Could you check a few things on this model? Use its own coordinates, in mm. Face numbers are marked on the shaded views. A direction names the side the tool comes from. Round coordinates to 2 decimals unless told otherwise and drop trailing zeros. Loops run counter-clockwise (first coordinate to the right, second up) from the corner with the lowest first, then second, coordinate; pieces in that order, holes last. Notation, with made-up numbers: (65.25, 50) -> (90.25, 50) arc R29 cw to (90.25, 71) -> close; hole circle Ø4 at (83, 85.25). An arc over 180 degrees is marked (long way). One line per item, written item: value.
Autodesk Inventor part; units mm, degrees
ref_plane "YZ Plane" through (0, 0, 0) normal (1, 0, 0) x (0, 1, 0)
ref_plane "XZ Plane" through (0, 0, 0) normal (0, 1, 0) x (-1, 0, 0)
ref_plane "XY Plane" through (0, 0, 0) normal (0, 0, 1) x (1, 0, 0)
sketch "Sketch1" plane through (0, 0, 0) normal (0, 1, 0) x (-1, 0, 0)
  line L0 (22.75, -10.36) -> (7.75, -10.36)
  line L1 (7.75, -10.36) -> (-0.1031, 0)
  circle A0 centre (4.34, -10.36) radius 1
  line L2 (22.75, 10.36) -> (7.75, 10.36)
  circle A1 centre (12.64, 0) radius 9.6 construction
  line L3 (22.75, 12.36) -> (22.75, -12.36)
  circle A2 centre (4.34, 10.36) radius 1
  line L4 (7.75, 10.36) -> (-0.1031, 0)
  line L5 (26.25, 17) -> (26.25, -17)
  line L6 (22.75, -12.36) -> (-22.75, -12.36)
  line L7 (22.75, 0) -> (-22.75, 0) construction
  line L8 (26.25, -17) -> (-28.75, -17)
  line L9 (26.25, -17) -> (-28.75, 17) construction
  line L10 (-28.75, -17) -> (26.25, 17) construction
  line L11 (-22.75, 12.36) -> (22.75, 12.36)
  line L12 (-28.75, 17) -> (26.25, 17)
  line L13 (-28.75, -17) -> (-28.75, 17)
  circle A3 centre (-16.36, 10.25) radius 1
  line L14 (-22.75, -12.36) -> (-22.75, 12.36)
  circle A4 centre (-16.36, -10.25) radius 1
  point P0 (0, 0)
  point P1 (-1.25, 0)
  point P2 (0, 0)
  point P3 (22.75, -10.36)
  dimension "d0" = 55
  dimension "d1" = 34
  dimension "d2" = 45.5
  dimension "d3" = 24.72
  dimension "d4" = 2
  dimension "d6" = 18.41
  dimension "d7" = 20.5
  dimension "d8" = 19.2
  dimension "d9" = 10.11
  dimension "d10" = 13
  dimension "d11" = 15
  dimension "d12" = 3.5
  dimension "d13" = 2
  dimension "d14" = 3.41
  dimension "d51" = 20.7
extrude "Extrusion1" add sketch "Sketch1" along normal mid plane 1 contours L3 L6 L14 L11 L2 L4 L1 L0 | L5 L8 L13 L12
extrude "Extrusion2" add sketch "Sketch1" along normal blind 35 contours L5 L8 L13 L12
fillet "Fillet1" radius 3 8 edges at (1.25, -0.5, -17) (28.75, -0.5, 0) (1.25, -0.5, 17) (-26.25, -0.5, 0) (28.75, 17.25, -17) (28.75, 17.25, 17) (-26.25, 17.25, 17) (-26.25, 17.25, -17)
sketch "Sketch3" plane through (-23.25, 35, 17) normal (0, 0, 1) x (1, 0, 0)
  line L0 (46, -34.5) -> (46, 0)
  circle A0 centre (46, -28) radius 1.5
  line L1 (49, -32.5) -> (0, -32.5)
  circle A1 centre (46, -17) radius 1.5
  circle A2 centre (46, -6) radius 1.5
  circle A3 centre (30, -28) radius 1.5
  circle A4 centre (30, -17) radius 1.5
  circle A5 centre (30, -6) radius 1.5
  line L2 (52, -32.5) -> (52, 0)
  point P0 (23.25, -35)
  dimension "d20" = 3
  dimension "d23" = 11
  dimension "d26" = 16
  dimension "d29" = 4.5
  dimension "d37" = 6
hole "Hole1" at (22.75, 7, 17) at (6.75, 7, 17) at (6.75, 18, 17) at (22.75, 18, 17) at (22.75, 29, 17) at (6.75, 29, 17) direction (0, 0, -1) diameter 2.459 depth 3 tip angle 118 counterbore diameter 3.9 counterbore depth 1.8
properties part number "basket"
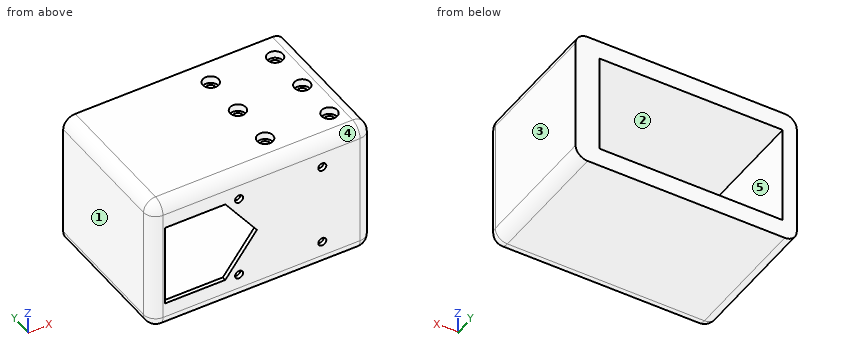
(1) If we section it at C-C, the plane x = -4: Please give me the cut outline in (y, z), then the cut area to 3 significant figures.
Recorded:
outline: (-0.5, -14) arc R3 ccw to (2.5, -17) -> (35, -17) -> (35, -12.36) -> (0.5, -12.36) -> (0.5, -11.3) -> (-0.5, -11.3) -> close; (-0.5, -9.42) -> (0.5, -9.42) -> (0.5, -5.41) -> (-0.5, -5.41) -> close; (-0.5, 5.41) -> (0.5, 5.41) -> (0.5, 9.42) -> (-0.5, 9.42) -> close; (-0.5, 11.3) -> (0.5, 11.3) -> (0.5, 12.36) -> (35, 12.36) -> (35, 17) -> (2.5, 17) arc R3 ccw to (-0.5, 14) -> close
area: 336 mm²
(2) If we section it at A-A, the plane x = -10: Please give me the cut outline in (y, z), then the cut area to 3 significant figures.
Recorded:
outline: (-0.5, -14) arc R3 ccw to (2.5, -17) -> (35, -17) -> (35, -12.36) -> (0.5, -12.36) -> (0.5, -10.36) -> (-0.5, -10.36) -> close; (-0.5, 10.36) -> (0.5, 10.36) -> (0.5, 12.36) -> (35, 12.36) -> (35, 17) -> (2.5, 17) arc R3 ccw to (-0.5, 14) -> close
area: 330 mm²
(3) Thinking about a two-plate mould opening in Z: for the marked faces 3, 4 and 5, which applies, released by +Z, released by -Z, zero draft, split by the parting line, or undercut?
Recorded:
face 3: zero draft
face 4: released by +Z
face 5: undercut
(4) I'm going to push a flat-ended pin straight in: pin 1 Ø3.5 at (x, y) = (22.75, 18) entering from +Z. Where does the tip first touch, or does it pass through?
Recorded:
pin 1: z = 15.2
(5) If we section it at B-B, the plane y = 10.5: Please give me the cut outline in (x, z).
Recorded:
outline: (-26.25, -14) arc R3 ccw to (-23.25, -17) -> (25.75, -17) arc R3 ccw to (28.75, -14) -> (28.75, 14) arc R3 ccw to (25.75, 17) -> (-23.25, 17) arc R3 ccw to (-26.25, 14) -> close; hole (-22.75, -12.36) -> (22.75, -12.36) -> (22.75, 12.36) -> (-22.75, 12.36) -> close
(6) For the marked faces 1 and 2, which set-ups out of +Z, -Z, +X, -X, +Y, -Y let a thin tool reach every point of the face, with its end or its side?
Recorded:
face 1: +Z, -Z, -X, +Y, -Y
face 2: +Y
(7) If I drill on L1, parallel to X at y = 29, z = 14; L2, parallel to Z at x = -18.5, y = 6.5; L3, parallel to X at y = 29, z = 14.8, over which ranges is the centre line in solid material (lowest first)?
Recorded:
L1: -26.25 to 5.52, 7.98 to 21.52, 23.98 to 28.75
L2: -17 to -12.36, 12.36 to 17
L3: -26.14 to 5.52, 7.98 to 21.52, 23.98 to 28.64
(8) If we section it at D-D, the plane x = 16: Please give me the cut outline in (y, z), then the cut area to 3 significant figures.
Recorded:
outline: (-0.5, -14) arc R3 ccw to (2.5, -17) -> (35, -17) -> (35, -12.36) -> (0.5, -12.36) -> (0.5, -11.18) -> (-0.5, -11.18) -> close; (-0.5, -9.32) -> (0.5, -9.32) -> (0.5, 9.32) -> (-0.5, 9.32) -> close; (-0.5, 11.18) -> (0.5, 11.18) -> (0.5, 12.36) -> (35, 12.36) -> (35, 17) -> (2.5, 17) arc R3 ccw to (-0.5, 14) -> close
area: 347 mm²
